For this review, take the finished solid that the model builds, in its own axes (mm). A direction names the side the tool comes from. Give positions to 0.01 mm unless a question says otherwise; leave off trailing zeros. Write each loop counter-clockwise with the first axis right and the second up, starting at its lowest first coordinate (ties: lowest second). Pieces come first, ordered by that corner, then holes.
1) Draft analysis for pull direction Z (two halves, no side actions). For faces 3 (the face through (46.011, 25, -30)), 4 (the face through (49, 15, -100)), 5 (the face through (100, 15, -49)), state which applies: pulls with the +Z half, pulls with the -Z half, needs draft (parallel to the pull), parting line crosses it, or undercut.
2) We need section C-C on y = 27.25. Give the boundary of the cut face in (x, z), and give its area (3 significant figures).
3) We need section B-B on z = -22. Give the boundary of the cut face in (x, y), and give its area (3 significant figures).
4) Machinability: for faces 1 (the face through (0, 15, -49)), 2 (the face through (27, 25, -9.374)), which of the approach directions +Z, -Z, +X, -X, +Y, -Y give a long, thin tool a straight path to every point of the face, cutting with its end or side? Answer none if there is none.
5) For P1, Ø11, axis at x = 28, y = 24, coming from the +Z side; P2, Ø12, axis at x = 24.5, z = -26.5, coming from the +Y side, all flat-tipped, find the tip position at first contact; note any pin that passes through.
6) Wall thickness on line 1 along Z through (x, y) = (19.5, 23); line 2 along X through (y, z) = (24, -40.5); line 3 along Y through (x, z) = (45.5, -39): over which ranges is each line inside the solid? List them lowest first.
7) We need section A-A on x = 24. Give the boundary of the cut face in (y, z).
from build123d import *

# Parameters (mm, degrees)
SKETCH1_W           = 100
SKETCH1_H           = 100
BOSS_EXTRUDE1_DEPTH = 30
SKETCH5_R           = 2
CUT_EXTRUDE1_DEPTH  = 31
SKETCH7_R           = 22.78996388
SKETCH7_W           = 37.683489423
SKETCH7_H           = 41.413312703
CUT_EXTRUDE2_DEPTH  = 10
FILLET1_R           = 3


with BuildPart() as part:
    # Sketch1 → Boss-Extrude1 (new body)
    with BuildSketch(Plane(origin=(0, 0, 0), x_dir=(1, 0, 0), z_dir=(0, 1, 0))):
        with Locations((50, 50)):
            Rectangle(SKETCH1_W, SKETCH1_H)
    extrude(amount=BOSS_EXTRUDE1_DEPTH)

    # Sketch5 → Cut-Extrude1 (cut, through all)
    with BuildSketch(Plane(origin=(0, 30, 0), x_dir=(1, 0, 0), z_dir=(0, 1, 0))):
        with Locations((16.384313545, 87.323198024)):
            Circle(SKETCH5_R)
    extrude(amount=-CUT_EXTRUDE1_DEPTH, mode=Mode.SUBTRACT)

    # Sketch7 → Cut-Extrude2 (cut)
    with BuildSketch(Plane(origin=(0, 30, 0), x_dir=(1, 0, 0), z_dir=(0, 1, 0))):
        with Locations((72.084640228, 73.225170758)):
            Circle(SKETCH7_R)
        with Locations((27.16963915, 30.080771209)):
            Rectangle(SKETCH7_W, SKETCH7_H)
    extrude(amount=-CUT_EXTRUDE2_DEPTH, mode=Mode.SUBTRACT)

    # Fillet1
    fillet1_edges = [part.edges().sort_by_distance(p)[0] for p in [
        (8.327894438, 25, -9.374114858),
        (8.327894438, 25, -50.787427561),
        (46.011383861, 25, -50.787427561),
        (46.011383861, 25, -9.374114858),
    ]]
    fillet(fillet1_edges, radius=FILLET1_R)


solid = part.part
Results list:
1. face 3: undercut
1. face 4: pulls with the -Z half
1. face 5: needs draft
2. outline: (0, -100) - (100, -100) - (100, 0) - (0, 0) - close; hole (8.33, -47.79) arc R3 ccw to (11.33, -50.79) - (43.01, -50.79) arc R3 ccw to (46.01, -47.79) - (46.01, -12.37) arc R3 ccw to (43.01, -9.37) - (11.33, -9.37) arc R3 ccw to (8.33, -12.37) - close; hole circle Ø4 at (16.38, -87.32); hole circle Ø45.58 at (72.08, -73.23)
2. area: 6,800 mm2
3. outline: (0, 0) - (100, 0) - (100, 30) - (46.01, 30) - (46.01, 20) - (8.33, 20) - (8.33, 30) - (0, 30) - close
3. area: 2,620 mm2
4. face 1: +Z, -Z, -X, +Y, -Y
4. face 2: +Y
5. P1: stops at z = 0
5. P2: stops at y = 20
6. line 1: z = -100 to -50.79, -9.37 to 0
6. line 2: x = 0 to 8.33, 46.01 to 100
6. line 3: y = 0 to 20
7. outline: (0, -100) - (30, -100) - (30, -50.79) - (20, -50.79) - (20, -9.37) - (30, -9.37) - (30, 0) - (0, 0) - close
